Read the model definition and answer for the solid it produces. Units are mm, in the model's axes. Face numbers are marked on the shaded views. A direction names the side the tool comes from. Give positions to 0.01 mm unless a question says otherwise; leave off trailing zeros. Order: outer loops, then holes, each group sorted by start corner. A loop starts at its lowest first (then second) coordinate and runs counter-clockwise, first axis right, second up. Notation, with made-up numbers: (59.25, 43) -> (65.25, 43) arc R16 cw to (65.25, 56) -> close; hole circle Ø8 at (5, 18). An arc over 180 degrees is marked (long way). Answer as CSV lines item,"result". Start each with the question number.
1) Find section C-C (x = 17). Determine the outline of the cut face in (y, z), and give its area (3 significant figures).
2) The mould has two halves that part along Y. Classify the marked faces 6, 7, 8 and 9: +Y half, -Y half, draft (parallel to the pull), parting line (faces both ways), or undercut.
3) Find section D-D (z = -9). Determine the outline of the cut face in (x, y).
4) For the marked faces 1, 2, 3, 4 and 5, determine the directions among +Z, -Z, +X, -X, +Y, -Y from which every point of the face is accessible in a straight line to the end or side of a thin tool.
5) Straight lines are drawn through the part: L1, parallel to Z at x = 24.75, y = 30.1; L2, parallel to Y at x = 2, z = 4; L3, parallel to X at y = 29.9, z = -5. For each, find the intervals that lie inside material, in ascending order. Write a range as from..to.
6) Find section A-A (x = 24.75). Determine the outline of the cut face in (y, z).
7) Find section B-B (z = 5). Determine the outline of the cut face in (x, y), and give its area (3 significant figures).
8) Flat-ended cylindrical pins translate along their axes: pin 1 Ø3 at (y, z) = (35, -2) entering from -X; pin 2 Ø1.5 at (x, y) = (22, 26.5) entering from -Z; pin 3 Ø1.1 at (x, y) = (23, 32) entering from +Z; pin 4 Ø6 at (x, z) = (-24, -5) entering from +Y. Find the tip coordinate at first contact, or state that the pin passes through.
Autodesk Inventor part; units mm, degrees
ref_plane "YZ Plane" through (0, 0, 0) normal (1, 0, 0) x (0, 1, 0)
ref_plane "XZ Plane" through (0, 0, 0) normal (0, 1, 0) x (-1, 0, 0)
ref_plane "XY Plane" through (0, 0, 0) normal (0, 0, 1) x (1, 0, 0)
sketch "Sketch1" plane through (0, 0, 0) normal (0, 0, 1) x (1, 0, 0)
  line L0 (-20, 0) -> (20, 0)
  line L1 (20, 0) -> (20, 28.7)
  line L2 (20, 28.7) -> (27.4, 28.7)
  line L3 (27.4, 28.7) -> (27.4, 31.2)
  line L4 (27.4, 31.2) -> (20, 31.2)
  line L5 (20, 31.2) -> (20, 37)
  line L6 (20, 37) -> (-20, 37)
  line L7 (-20, 37) -> (-20, 31.2)
  line L8 (-20, 31.2) -> (-27.4, 31.2)
  line L9 (-27.4, 31.2) -> (-27.4, 28.7)
  line L10 (-27.4, 28.7) -> (-20, 28.7)
  line L11 (-20, 28.7) -> (-20, 0)
  point P0 (0, 0)
  point P1 (0, 0)
  dimension "d0" = 40
  dimension "d1" = 28.7
  dimension "d2" = 7.4
  dimension "d3" = 2.5
  dimension "d4" = 5.8
  dimension "d5" = 7.4
extrude "Extrusion1" add sketch "Sketch1" along normal mid plane 20
sketch "Sketch4" plane through (0, 0, 0) normal (0, 0, 1) x (1, 0, 0)
  line L0 (20, 37) -> (-20, 37)
  line L1 (12.5, 37) -> (12.5, 41.4)
  line L2 (12.5, 41.4) -> (20.1, 41.4)
  line L3 (20.1, 41.4) -> (20.1, 44.4)
  line L4 (20.1, 44.4) -> (12.5, 44.4)
  line L5 (12.5, 44.4) -> (12.5, 44.8)
  line L6 (12.5, 44.8) -> (9.7, 44.8)
  line L7 (12.5, 37) -> (9.7, 37)
  line L8 (9.7, 44.8) -> (9.7, 37)
  point P0 (0, 0)
  point P1 (0, 37)
  dimension "d10" = 9.7
  dimension "d11" = 0.4
  dimension "d12" = 10.4
  dimension "d13" = 2.8
  dimension "d14" = 4.4
  dimension "d15" = 3
revolve "Revolution1" add sketch "Sketch4" angle 360 about axis through (9.7, 44.8, 0) along (0, -1, 0)
sketch "Sketch5" plane through (-27.4, 31.2, 10) normal (0, 1, 0) x (1, 0, 0)
  circle A0 centre (2.65, 15) radius 2
  line L0 (0, 20) -> (0, 0)
  line L1 (7.4, 0) -> (0, 0)
  line L2 (7.4, 20) -> (7.4, 0)
  line L3 (0, 20) -> (7.4, 20)
  line L4 (47.4, 20) -> (47.4, 0)
  line L5 (54.8, 0) -> (47.4, 0)
  line L6 (54.8, 20) -> (54.8, 0)
  line L7 (47.4, 20) -> (54.8, 20)
  line L8 (7.4, 20) -> (47.4, 20)
  line L9 (27.4, 20) -> (27.4, 0) construction
  line L10 (7.4, 0) -> (47.4, 0)
  line L11 (0, 20) -> (0, 0)
  line L12 (0, 10) -> (54.8, 10) construction
  line L13 (54.8, 20) -> (54.8, 0)
  circle A1 centre (2.65, 5) radius 2
  circle A2 centre (52.15, 15) radius 2
  circle A3 centre (52.15, 5) radius 2
  line L14 (7.4, 0) -> (7.4, 20)
  line L15 (7.4, 10.75) -> (0, 10.75)
  line L16 (0, 10.75) -> (0, 9.25)
  line L17 (0, 9.25) -> (7.4, 9.25)
  line L18 (7.4, 9.25) -> (7.4, 10.75)
  line L19 (47.4, 10.75) -> (54.8, 10.75)
  line L20 (54.8, 10.75) -> (54.8, 9.25)
  line L21 (54.8, 9.25) -> (47.4, 9.25)
  line L22 (47.4, 9.25) -> (47.4, 10.75)
  point P0 (27.4, 10)
  dimension "d17" = 4
  dimension "d18" = 10
  dimension "d19" = 49.5
  dimension "d22" = 7.4
  dimension "d23" = 1.5
extrude "Extrusion2" cut sketch "Sketch5" against normal up to next contours A0 | A1 | A2 | A3
extrude "Extrusion3" add sketch "Sketch5" along normal blind 1 contours L15 L2 L17 L0 | L19 L6 L21 L4
sketch "Sketch6" plane through (-20, 0, 10) normal (0, -1, 0) x (1, 0, 0)
  line L0 (0, 0) -> (0, -20) construction
  line L1 (0, -10) -> (40, -10) construction
  line L2 (40, -20) -> (40, 0) construction
  line L3 (40, 0) -> (0, 0) construction
  line L4 (20, 0) -> (20, -20) construction
  line L5 (0, -20) -> (40, -20) construction
  line L6 (40, 0) -> (0, 0) construction
  line L7 (0, 0) -> (0, -20) construction
  line L8 (0, -20) -> (40, -20) construction
  line L9 (40, -20) -> (40, 0) construction
  circle A0 centre (29.7, -10) radius 2.8
  circle A1 centre (-4.75, -5) radius 2
  circle A2 centre (-4.75, -15) radius 2
  circle A3 centre (44.75, -15) radius 2
  circle A4 centre (44.75, -5) radius 2
  line L10 (-7.4, -10.75) -> (0, -10.75)
  line L11 (0, -9.25) -> (-7.4, -9.25)
  line L12 (40, -10.75) -> (47.4, -10.75)
  line L13 (47.4, -9.25) -> (40, -9.25)
  line L14 (40, -20) -> (40, 0)
  line L15 (47.4, -20) -> (47.4, 0)
  line L16 (40, 0) -> (47.4, 0)
  circle A5 centre (44.75, -15) radius 2
  circle A6 centre (44.75, -5) radius 2
  line L17 (47.4, -20) -> (47.4, 0)
  line L18 (40, 0) -> (47.4, 0)
  line L19 (40, -20) -> (40, 0)
  line L20 (47.4, -20) -> (40, -20)
  circle A7 centre (-4.75, -15) radius 2
  circle A8 centre (-4.75, -5) radius 2
  line L21 (0, -20) -> (0, 0)
  line L22 (-7.4, 0) -> (0, 0)
  line L23 (-7.4, -20) -> (-7.4, 0)
  line L24 (0, -20) -> (-7.4, -20)
  point P0 (20, -10)
properties part number "feedback_servo"
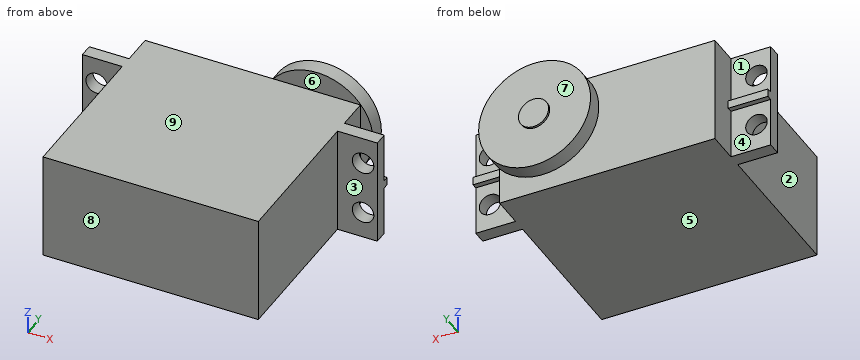
Findings below:
1,outline,"(0, -10) -> (37, -10) -> (37, 10) -> (0, 10) -> close; (41.4, -7.41) -> (44.4, -7.41) -> (44.4, 7.41) -> (41.4, 7.41) -> close"
1,area,"784 mm²"
2,face 6,"undercut"
2,face 7,"+Y half"
2,face 8,"-Y half"
2,face 9,"draft"
3,outline,"(-27.4, 28.7) -> (-20, 28.7) -> (-20, 0) -> (20, 0) -> (20, 28.7) -> (27.4, 28.7) -> (27.4, 31.2) -> (20, 31.2) -> (20, 37) -> (-20, 37) -> (-20, 31.2) -> (-27.4, 31.2) -> close; (4.49, 41.4) -> (14.91, 41.4) -> (14.91, 44.4) -> (4.49, 44.4) -> close"
4,face 1,"+Z, -X, +Y"
4,face 2,"+Z, -Z, -X, -Y"
4,face 3,"+Z, -Z, +X, -Y"
4,face 4,"-Z, -X, +Y"
4,face 5,"-Z, +X, -X, -Y"
5,L1,"-10..-7, -3..3, 7..10"
5,L2,"0..37, 41.4..44.4"
5,L3,"-27.4..-26.75, -22.75..22.75, 26.75..27.4"
6,outline,"(28.7, -10) -> (31.2, -10) -> (31.2, -7) -> (28.7, -7) -> close; (28.7, -3) -> (31.2, -3) -> (31.2, -0.75) -> (32.2, -0.75) -> (32.2, 0.75) -> (31.2, 0.75) -> (31.2, 3) -> (28.7, 3) -> close; (28.7, 7) -> (31.2, 7) -> (31.2, 10) -> (28.7, 10) -> close"
7,outline,"(-27.4, 28.7) -> (-26.75, 28.7) -> (-26.75, 31.2) -> (-27.4, 31.2) -> close; (-22.75, 28.7) -> (-20, 28.7) -> (-20, 0) -> (20, 0) -> (20, 28.7) -> (22.75, 28.7) -> (22.75, 31.2) -> (20, 31.2) -> (20, 37) -> (-20, 37) -> (-20, 31.2) -> (-22.75, 31.2) -> close; (0.58, 41.4) -> (18.82, 41.4) -> (18.82, 44.4) -> (0.58, 44.4) -> close; (26.75, 28.7) -> (27.4, 28.7) -> (27.4, 31.2) -> (26.75, 31.2) -> close"
7,area,"1,550 mm²"
8,pin 1,"x = -20"
8,pin 2,"through"
8,pin 3,"z = 0.75"
8,pin 4,"y = 31.2"
